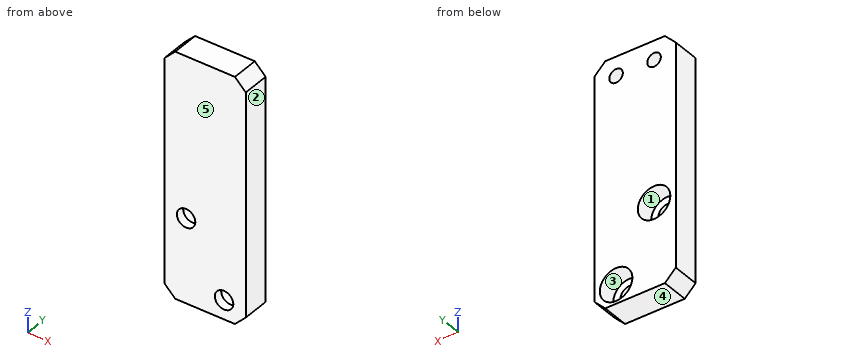
```python
from build123d import *

# Parameters (mm, degrees)
SKETCH1_W                                            = 15
SKETCH1_H                                            = 45
BOSS_EXTRUDE1_DEPTH                                  = 5
M3_TAPPED_HOLE1_D                                    = 2.5
M3_TAPPED_HOLE1_DEPTH                                = 4
M3_TAPPED_HOLE1_TIP                                  = 0.751075774
CBORE_FOR_M3_HEXAGON_SOCKET_HEAD_CAP_SCR_D           = 3.4
CBORE_FOR_M3_HEXAGON_SOCKET_HEAD_CAP_SCR_CBORE_D     = 6
CBORE_FOR_M3_HEXAGON_SOCKET_HEAD_CAP_SCR_CBORE_DEPTH = 3.4
CHAMFER1_SIZE                                        = 2


with BuildPart() as part:
    # Sketch1 → Boss-Extrude1 (new body)
    with BuildSketch(Plane(origin=(0, 0, 0), x_dir=(1, 0, 0), z_dir=(0, 1, 0))):
        Rectangle(SKETCH1_W, SKETCH1_H)
    extrude(amount=BOSS_EXTRUDE1_DEPTH)

    # M3 Tapped Hole1
    with Locations(Plane(origin=(0, 5, 0), x_dir=(1, 0, 0), z_dir=(0, 1, 0))):
        with Locations((-3.5, -19), (3.5, -19)):
            Hole(M3_TAPPED_HOLE1_D / 2, depth=M3_TAPPED_HOLE1_DEPTH)
            with Locations((0, 0, -(M3_TAPPED_HOLE1_DEPTH + M3_TAPPED_HOLE1_TIP / 2))):  # 118° drill point
                Cone(0, M3_TAPPED_HOLE1_D / 2, M3_TAPPED_HOLE1_TIP, mode=Mode.SUBTRACT)

    # CBORE for M3 Hexagon socket head cap screws1 (through all)
    with Locations(Plane(origin=(0, 5, 0), x_dir=(1, 0, 0), z_dir=(0, 1, 0))):
        with Locations((3.5, 19), (-3.5, 7)):
            CounterBoreHole(CBORE_FOR_M3_HEXAGON_SOCKET_HEAD_CAP_SCR_D / 2, CBORE_FOR_M3_HEXAGON_SOCKET_HEAD_CAP_SCR_CBORE_D / 2, CBORE_FOR_M3_HEXAGON_SOCKET_HEAD_CAP_SCR_CBORE_DEPTH)

    # Chamfer1
    chamfer1_edges = [part.edges().sort_by_distance(p)[0] for p in [
        (7.5, 2.5, 22.5),
        (-7.5, 2.5, 22.5),
        (-7.5, 2.5, -22.5),
        (7.5, 2.5, -22.5),
    ]]
    chamfer(chamfer1_edges, length=CHAMFER1_SIZE)


solid = part.part
```
The listing builds one solid part. Answer for the finished solid, in the listing's coordinates (mm). Face numbers are marked on the shaded views. A direction names the side the tool comes from. Give positions to 0.01 mm unless a question says otherwise; leave off trailing zeros. Loops run counter-clockwise (first coordinate to the right, second up) from the corner with the lowest first, then second, coordinate; pieces in that order, holes last. Notation, with made-up numbers: (33.5, -40) - (77.5, -40) arc R11 cw to (77.5, -31) - close; hole circle Ø2 at (76.5, -25). An arc over 180 degrees is marked (long way). Return JSON: item names as keys, results as strings. Group by question number.
1. Which of the six approach directions +Z, -Z, +X, -X, +Y, -Y give full straight-line access (tool end or side, diameter ignored) to the marked faces 1 and 2?
2. Find section B-B (y = 2.95). Write down the section's boundary in (x, z).
3. Straight lines are drawn through the part: line 1 (Z direction, x = -3.5, y = 1.2); line 2 (Z direction, x = 3.5, y = 2.5); line 3 (X direction, y = 3.5, z = 19). For each, find the intervals that lie inside material, in ascending order. Write a range as [from, to].
4. Determine the mould class of the marked faces 3, 4 and 5 for opening direction Z: pulls with the +Z half, pulls with the -Z half, needs draft (parallel to the pull), parting line crosses it, or undercut.
5. Given pin 1 Ø3 at (x, z) = (4, -19) entering from +Y; pin 2 Ø2 at (x, z) = (-3.5, 19) entering from +Y, each flat-ended and moving along its own axis, determine where each tip first touches the part or whether it passes through.
6. Find section A-A (z = -7). Write down the section's boundary in (x, y).
Verdict:
{
 "1": {"face 1": "+Y", "face 2": "+Z, -Z, +X, +Y, -Y"},
 "2": {"outline": "(-7.5, -20.5) - (-5.5, -22.5) - (5.5, -22.5) - (7.5, -20.5) - (7.5, 20.5) - (5.5, 22.5) - (-5.5, 22.5) - (-7.5, 20.5) - close; hole circle Ø6 at (-3.5, -7); hole circle Ø2.5 at (-3.5, 19); hole circle Ø6 at (3.5, -19); hole circle Ø2.5 at (3.5, 19)"},
 "3": {"line 1": "z = [-22.5, -8.7], [-5.3, 17.75], [20.25, 22.5]", "line 2": "z = [-22.5, -22], [-16, 17.75], [20.25, 22.5]", "line 3": "x = [-7.5, -4.75], [-2.25, 2.25], [4.75, 7.5]"},
 "4": {"face 3": "undercut", "face 4": "pulls with the -Z half", "face 5": "needs draft"},
 "5": {"pin 1": "stops at y = 1.6", "pin 2": "stops at y = 0.85"},
 "6": {"outline": "(-7.5, 0) - (-5.2, 0) - (-5.2, 1.6) - (-6.5, 1.6) - (-6.5, 5) - (-7.5, 5) - close; (-1.8, 0) - (7.5, 0) - (7.5, 5) - (-0.5, 5) - (-0.5, 1.6) - (-1.8, 1.6) - close"}
}
